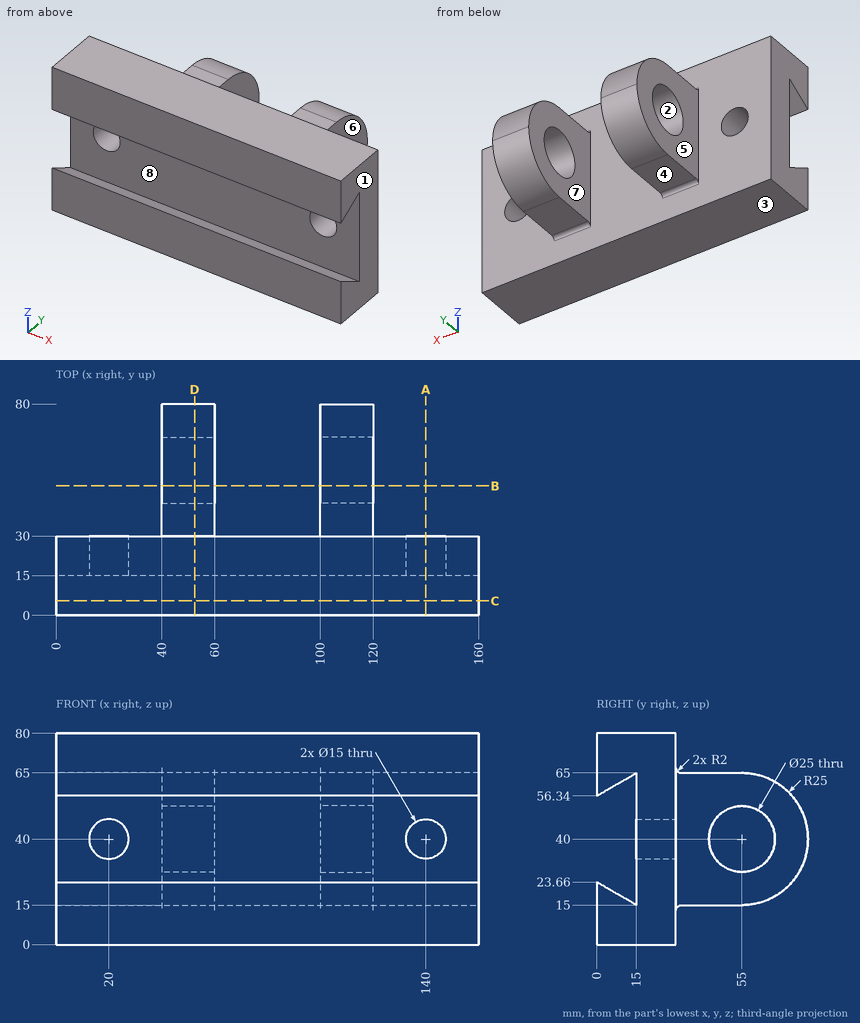
Geometry check sheet. Reference: drawing and pictorial views, mm from the part's lowest x, y, z. A direction names the side the tool comes from. Round coordinates to 2 decimals unless told otherwise and drop trailing zeros. Order: outer loops, then holes, each group sorted by start corner. A loop starts at its lowest first (then second) coordinate and runs counter-clockwise, first axis right, second up. Notation, with made-up numbers: (-7.5, 53.25) - (25.5, 53.25) arc R27 cw to (25.5, 71.25) - close; hole circle Ø7 at (83, 10). An arc over 180 degrees is marked (long way). One line per question, with ' | ' between items. Start each with the question number.
(1) Access from +Z, -Z, +X, -X, +Y, -Y to the whole of each face (thin tool, end or side, straight path). Record for the marked faces 4, 5, 6, 7 and 8.
(2) Sectioned sample at C-C on y = 5.5. Record the cut outline in (x, z) (1 decimal).
(3) Sectioned sample at B-B on y = 49. Record the cut outline in (x, z), and give its area (3 significant figures).
(4) Sectioned sample at A-A on x = 140. Record the cut outline in (y, z), and give its area (4 significant figures).
(5) Release check for a two-part mould opening along Z. For the marked faces 1, 2 and 3 record: released by +Z, released by -Z, zero draft, split by the parting line, or undercut.
(6) Depth check by flat-ended pin: pin 1 Ø15 at (y, z) = (45.5, 52.5) entering from +X; pin 2 Ø6 at (x, y) = (108.5, 48.5) entering from +Z; pin 3 Ø10 at (x, y) = (111, 47.5) entering from -Z. Enter the tip coordinate at first touch or a pass-through.
(7) Sectioned sample at D-D on x = 52.5. Record the cut outline in (y, z).
(8) Thickness scan on L1, parallel to X at y = 23.5, z = 40; L2, parallel to X at y = 57.5, z = 53; L3, parallel to Z at x = 105, y = 55. Record the ranges inside material, lowest first. Write a range as [from, to].
Conclusion:
1) face 4: -Z, +X, -X, +Y | face 5: +Z, -Z, -X, +Y | face 6: +Z, -Z, +X, +Y | face 7: +Z, -Z, +Y | face 8: +X, -X
2) outline: (0, 0) - (160, 0) - (160, 20.5) - (0, 20.5) - close; (0, 59.5) - (160, 59.5) - (160, 80) - (0, 80) - close
3) outline: (40, 15) - (60, 15) - (60, 29.03) - (40, 29.03) - close; (40, 50.97) - (60, 50.97) - (60, 65) - (40, 65) - close; (100, 15) - (120, 15) - (120, 29.03) - (100, 29.03) - close; (100, 50.97) - (120, 50.97) - (120, 65) - (100, 65) - close | area: 1,120 mm2
4) outline: (0, 0) - (30, 0) - (30, 32.5) - (15, 32.5) - (15, 15) - (0, 23.66) - close; (0, 56.34) - (15, 65) - (15, 47.5) - (30, 47.5) - (30, 80) - (0, 80) - close | area: 1,555 mm2
5) face 1: zero draft | face 2: undercut | face 3: released by -Z
6) pin 1: stops at x = 120 | pin 2: stops at z = 65 | pin 3: stops at z = 15
7) outline: (0, 0) - (30, 0) - (30, 13) arc R2 cw to (32, 15) - (55, 15) arc R25 ccw to (55, 65) - (32, 65) arc R2 cw to (30, 67) - (30, 80) - (0, 80) - (0, 56.34) - (15, 65) - (15, 15) - (0, 23.66) - close; hole circle Ø25 at (55, 40)
8) L1: x = [0, 12.5], [27.5, 132.5], [147.5, 160] | L2: x = [40, 60], [100, 120] | L3: z = [15, 27.5], [52.5, 65]
